Check sheet for the modelled part. Datum: model origin and axes. Units: mm. Give positions to 0.01 mm unless a question says otherwise; leave off trailing zeros. Write each loop counter-clockwise with the first axis right and the second up, starting at its lowest first coordinate (ties: lowest second). Pieces come first, ordered by that corner, then holes. Notation, with made-up numbers: (10, 50) -> (54, 50) arc R22 cw to (54, 83) -> close; hole circle Ø1 at (79, -35.75). An arc over 180 degrees is marked (long way). Answer as a JSON object with one key per item and string values.
from build123d import *

# Parameters (mm, degrees)
F1_DEPTH = 12.7
F2_R     = 3.365552
F2_R_2   = 3.520723
F2_R_3   = 3.514653
F2_R_4   = 3.746049
F2_R_5   = 3.497554
F2_R_6   = 3.892974
F2_R_7   = 3.939651
F2_R_8   = 10.370237
F2_R_9   = 10.264594
F2_R_10  = 10.264592
F2_R_11  = 11.303067
F3_DEPTH = 12.7


with BuildPart() as f1:
    # F0 (on Top) → F1 (new body, symmetric)
    with BuildSketch(Plane.XY):
        with BuildLine():
            ThreePointArc((12.079931, -75.236396), (57.995391, -49.426457), (76.2, 0))
            ThreePointArc((76.2, 0), (-57.995391, 49.426457), (12.079931, -75.236396))
        make_face()
        with BuildLine():
            ThreePointArc((-11.6058, -62.430405), (-44.890071, -44.912488), (-62.424602, -11.636967))
            Line((-62.424602, -11.636967), (-11.6058, -11.636967))
            Line((-11.6058, -11.636967), (-11.6058, -62.430405))
        make_face(mode=Mode.SUBTRACT)
        with BuildLine():
            Line((12.079931, -62.340398), (12.079931, -11.636967))
            Line((12.079931, -11.636967), (62.424602, -11.636967))
            ThreePointArc((62.424602, -11.636967), (45.060413, -44.741582), (12.079931, -62.340398))
        make_face(mode=Mode.SUBTRACT)
        with BuildLine():
            ThreePointArc((-62.430405, 11.605796), (-44.901282, 44.901279), (-11.6058, 62.430405))
            Line((-11.6058, 62.430405), (-11.6058, 11.605796))
            Line((-11.6058, 11.605796), (-62.430405, 11.605796))
        make_face(mode=Mode.SUBTRACT)
        with BuildLine():
            ThreePointArc((0, 12.7), (8.980256, 8.980256), (12.7, 0))
            ThreePointArc((12.7, 0), (8.980256, -8.980256), (0, -12.7))
            ThreePointArc((0, -12.7), (-8.980256, -8.980256), (-12.7, 0))
            ThreePointArc((-12.7, 0), (-8.980256, 8.980256), (0, 12.7))
        make_face(mode=Mode.SUBTRACT)
        with BuildLine():
            Line((12.079931, 11.605796), (12.079931, 62.340398))
            ThreePointArc((12.079931, 62.340398), (45.071582, 44.73033), (62.430405, 11.605796))
            Line((62.430405, 11.605796), (12.079931, 11.605796))
        make_face(mode=Mode.SUBTRACT)
    extrude(amount=F1_DEPTH, both=True)

    # F2 (on Top) → F3 (cut, symmetric)
    with BuildSketch(Plane.XY):
        with Locations((-39.48367, 31.044669)):
            Circle(F2_R)
        with Locations((-28.732972, 30.837925)):
            Circle(F2_R)
        Polygon((-25.63181, 61.229318), (-30.386927, 65.570951), (-32.867856, 58.955137), align=None)
        Polygon((-14.157661, 63.081107), (-15.914831, 68.672113), (-18.085646, 62.883273), align=None)
        Polygon((0, 62.883273), (-3.096693, 68.672113), (-5.267507, 62.883273), align=None)
        Polygon((9.721447, 69.292344), (6.000051, 62.883273), (13.442842, 62.883273), align=None)
        Polygon((30.809354, 57.094436), (27.708191, 66.191182), (20.265399, 60.815834), align=None)
        with Locations((25.222793, 32.252096)):
            Circle(F2_R_2)
        with Locations((38.661163, 32.045349)):
            Circle(F2_R_3)
        with Locations((-37.420698, -32.44324)):
            Circle(F2_R_4)
        with Locations((-26.049767, -32.44324)):
            Circle(F2_R_5)
        with Locations((20.674419, -34.583465)):
            Circle(F2_R_6)
        with Locations((34.112792, -34.583465)):
            Circle(F2_R_7)
        with Locations((37.213955, 0)):
            Circle(F2_R_8)
        with Locations((-42.796046, 0)):
            Circle(F2_R_9)
        with Locations((0, 35.766747)):
            Circle(F2_R_10)
        with Locations((0, -43.209538)):
            Circle(F2_R_11)
    extrude(amount=F3_DEPTH, both=True, mode=Mode.SUBTRACT)


solid = f1.part
1. Mould release check, pull along X, two halves, no side actions. Record for faces 1 (the face through (-4.167, 65.818, -0.178)), 2 (the face through (5, 12, -12.7)): released by +X, released by -X, zero draft, split by the parting line, or undercut.
Determined:
{"face 1": "undercut", "face 2": "zero draft"}
2. Go/stop test with flat-tipped pins: P1, Ø18.5, axis at x = 37.21, y = 0, coming from the +Z side; P2, Ø7.5, axis at x = -37, z = 2, coming from the +Y side; P3, Ø12.5, axis at x = 33.5, z = 2.5, coming from the +Y side; P4, Ø2, axis at x = -13.5, y = -12.5, coming from the +Z side. Record where each tip stops, or that it passes through.
Determined:
{"P1": "through", "P2": "y = 68.56", "P3": "y = 71.16", "P4": "z = 12.7"}
3. Sectioned sample at C-C, the plane y = -47. Enter the section's corners in (x, z).
Determined:
{"outline": "(-59.98, -12.7) -> (-42.7, -12.7) -> (-42.7, 12.7) -> (-59.98, 12.7) -> close; (-11.61, -12.7) -> (-10.65, -12.7) -> (-10.65, 12.7) -> (-11.61, 12.7) -> close; (10.65, -12.7) -> (12.08, -12.7) -> (12.08, 12.7) -> (10.65, 12.7) -> close; (42.7, -12.7) -> (59.98, -12.7) -> (59.98, 12.7) -> (42.7, 12.7) -> close"}
4. Scan lines: L1, parallel to X at y = 31, z = 3.5; L2, parallel to X at y = 45, z = -0.5; L3, parallel to Y at x = -56, z = -8.75. Record each from-to range of solid material in increasing order. Write a range as [from, to].
Determined:
{"L1": "[-69.61, -55.42], [-11.61, -9.09], [9.09, 12.08], [55.42, 69.61]", "L2": "[-61.49, -44.8], [-11.61, -4.48], [4.48, 12.08], [44.8, 61.49]", "L3": "[-51.68, -29.94], [-11.64, 11.61], [29.94, 51.68]"}
5. Sectioned sample at B-B, the plane z = 10.25. State how many separate pieces and enclosed holes the cut face has, plus the area to 3 significant figures.
Determined:
{"separate pieces": "1", "enclosed holes": "14", "area": "8,930 mm^2"}
6. Sectioned sample at A-A, the plane y = 8. Enter the section's corners in (x, z), plus the area to 3 significant figures.
Determined:
{"outline": "(-75.78, -12.7) -> (-49.23, -12.7) -> (-49.23, 12.7) -> (-75.78, 12.7) -> close; (-36.36, -12.7) -> (-9.86, -12.7) -> (-9.86, 12.7) -> (-36.36, 12.7) -> close; (9.86, -12.7) -> (30.62, -12.7) -> (30.62, 12.7) -> (9.86, 12.7) -> close; (43.81, -12.7) -> (75.78, -12.7) -> (75.78, 12.7) -> (43.81, 12.7) -> close", "area": "2,690 mm^2"}
